```python
from build123d import *

# Parameters (mm, degrees)
PAD015_DEPTH            = 17
SKETCH026_R             = 1.6
POCKET011_DEPTH         = 5
POCKET012_DEPTH         = 5
FILLET004_R             = 1
CHAMFER002_SIZE         = 2
CHAMFER003_SIZE         = 1
PAD014_DEPTH            = 7
FILLET003_R             = 1
FILLET002_R             = 0.4
BODY006_ROLL_ANGLE      = -90
BODY006_PLACEMENT_ANGLE = 180


with BuildPart() as obj1:
    # Sketch027 → Pad015 (new body)
    with BuildSketch(Plane.XY):
        Polygon((-2, -24.6), (-2, -2), (-13, -2), (-13, 0), (0, 0), (0, -22.6), (18.4, -22.6), (18.4, 3.4), (20.4, 3.4), (20.4, -24.6), align=None)
    extrude(amount=PAD015_DEPTH)

    # Sketch026 (on Face2 of Pad015) → Pocket011 (cut)
    with BuildSketch(Plane.XZ.offset(2)):
        with Locations((-9, 3.655766)):
            Circle(SKETCH026_R)
        with Locations((-9, 12.077909)):
            Circle(SKETCH026_R)
    extrude(amount=-POCKET011_DEPTH, mode=Mode.SUBTRACT)

    # Sketch025 → Pocket012 (cut)
    with BuildSketch(Plane(origin=(18.4, 0, 0), x_dir=(0, -1, 0), z_dir=(-1, 0, 0))):
        with BuildLine():
            ThreePointArc((9.9528471273, 16.0383040886), (11.1, 12.4), (12.2471528727, 16.0383040886))
            Line((11.1, 16.8415491775), (12.2471528727, 16.0383040886))
            Line((9.9528471273, 16.0383040886), (11.1, 16.8415491775))
        make_face()
    extrude(amount=-POCKET012_DEPTH, mode=Mode.SUBTRACT)

    # Fillet004
    fillet004_edges = [obj1.edges().sort_by_distance(p)[0] for p in [
        (-2, -24.6, 8.5),
        (20.4, -24.6, 8.5),
    ]]
    fillet(fillet004_edges, radius=FILLET004_R)

    # Chamfer002
    chamfer002_edges = [obj1.edges().sort_by_distance(p)[0] for p in [
        (-13, -1, 17),
        (-13, -1, 0),
    ]]
    chamfer(chamfer002_edges, length=CHAMFER002_SIZE)

    # Chamfer003
    chamfer003_edges = [obj1.edges().sort_by_distance(p)[0] for p in [
        (20.4, 3.4, 8.5),
    ]]
    chamfer(chamfer003_edges, length=CHAMFER003_SIZE)

    # Sketch028 (on Face1 of Chamfer003) → Pad014 (join)
    with BuildSketch(Plane(origin=(0, 0, 0), x_dir=(1, 0, 0), z_dir=(0, 0, -1))):
        Polygon((13.8, 24.6), (12.4, 24.6), (12.4, 26.8), (8, 26.8), (8, 25.6), (6.6, 25.6), (6.6, 28.2), (13.8, 28.2), align=None)
    extrude(amount=-PAD014_DEPTH)

    # Fillet003
    fillet003_edges = [obj1.edges().sort_by_distance(p)[0] for p in [
        (12.4, -24.6, 3.5),
        (13.8, -24.6, 3.5),
    ]]
    fillet(fillet003_edges, radius=FILLET003_R)

    # Fillet002
    fillet002_edges = [obj1.edges().sort_by_distance(p)[0] for p in [
        (13.8, -28.2, 3.5),
        (6.6, -28.2, 3.5),
        (6.6, -25.6, 3.5),
        (12.4, -26.8, 3.5),
        (8, -26.8, 3.5),
        (8, -25.6, 3.5),
    ]]
    fillet(fillet002_edges, radius=FILLET002_R)


with BuildPart() as obj1_1:
    # Body006 roll: moved
    add(obj1.part.rotate(Axis((0, 0, 0), (1, 0, 0)), BODY006_ROLL_ANGLE))


with BuildPart() as obj1_2:
    # Body006 placement: moved
    add(obj1_1.part.moved(Location((-26.5, 36.8, 2.5))).rotate(Axis((-26.5, 36.8, 2.5), (0, 0, 1)), BODY006_PLACEMENT_ANGLE))


with BuildPart() as part_mirroring001:
    # Part__Mirroring001: instance of obj1
    add(obj1_2.part.mirror(Plane(origin=(0, 0, 0), x_dir=(0, -1, 0), z_dir=(1, 0, 0))))


solid = part_mirroring001.part
```
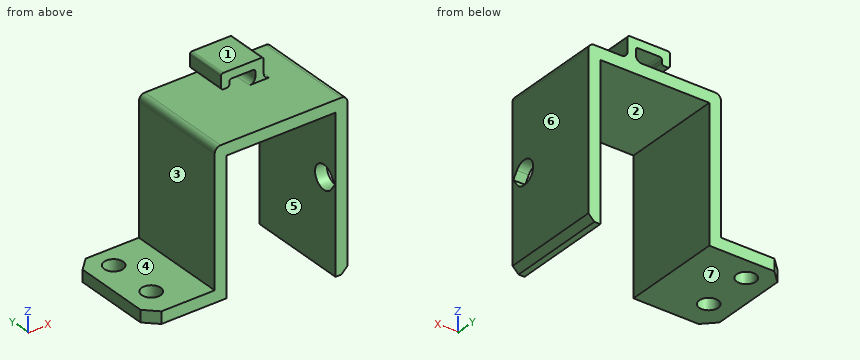
CAD build for the part. Positions are in the model's coordinates, mm. Face numbers are marked on the shaded views. A direction names the side the tool comes from. Coordinates: 2 decimals unless noted, no trailing zeros. Write each loop counter-clockwise with the first axis right and the second up, starting at its lowest first coordinate (ties: lowest second). Pieces come first, ordered by that corner, then holes. Notation, with made-up numbers: (51.5, 74) -> (83.5, 74) arc R35 ccw to (83.5, 110) -> close; hole circle Ø8 at (71, 84.25). An arc over 180 degrees is marked (long way). Return JSON: item names as keys, results as strings. Group by question number.
Q1. Cut at A-A, the plane x = 17.5. Give the cut face in (y, z), then the cut area to 3 significant figures.
Q2. Which spindle directions (+Z, -Z, +X, -X, +Y, -Y) get a long thin tool onto all of the face, cutting with end or side? Do the marked faces 4, 5, 6 and 7. Say none if no direction does.
Q3. Cut at C-C, the plane z = 16. Give the cut face in (x, y).
Q4. Cut at B-B, the plane y = 22.4. Give the cut face in (x, z), then the cut area to 3 significant figures.
Q5. Pull direction X, two halves, no side cores. Call the marked faces 1, 2 and 3: released by +X, released by -X, zero draft, split by the parting line, or undercut.
Q6. Flat gauge pins, fed straight in: pin 1 (5 mm diameter, centred on x = 31.5, y = 30.5, fed in from -Z); pin 2 (0.7 mm diameter, centred on y = 32, z = 29, fed in from +X); pin 3 (5 mm diameter, centred on x = 20.5, y = 29.5, fed in from +Z). Where does each tip first touch, or does it go through?
Q7. Drill centre lines: line 1 (X direction, y = 34.25, z = 15.5); line 2 (Y direction, x = 17, z = 3); line 3 (Z direction, x = 36.5, y = 32.25). Where is each one in solid material? Low to high.
Returned:
{
 "1": {"outline": "(19.8, 2.5) -> (23.12, 2.5) -> (23.12, 4.5) -> (19.8, 4.5) -> close; (26.32, 2.5) -> (31.54, 2.5) -> (31.54, 4.5) -> (26.32, 4.5) -> close; (34.74, 2.5) -> (36.8, 2.5) -> (36.8, 4.5) -> (34.74, 4.5) -> close", "area": "21.2 mm2"},
 "2": {"face 4": "+Z, -X, +Y, -Y", "face 5": "-Z, +Y, -Y", "face 6": "+Z, -Z, +X, +Y, -Y", "face 7": "-Z, -X, +Y, -Y"},
 "3": {"outline": "(24.5, 19.8) -> (26.5, 19.8) -> (26.5, 36.8) -> (24.5, 36.8) -> close; (44.9, 19.8) -> (46.9, 19.8) -> (46.9, 36.8) -> (44.9, 36.8) -> close"},
 "4": {"outline": "(13.5, 2.5) -> (26.5, 2.5) -> (26.5, 25.1) -> (44.9, 25.1) -> (44.9, 15.6) -> (46.9, 15.6) -> (46.9, 26.1) arc R1 ccw to (45.9, 27.1) -> (25.5, 27.1) arc R1 ccw to (24.5, 26.1) -> (24.5, 4.5) -> (13.5, 4.5) -> close; (44.9, -0.9) -> (45.9, -0.9) -> (46.9, 0.1) -> (46.9, 11.6) -> (44.9, 11.6) -> close", "area": "155 mm2"},
 "5": {"face 1": "zero draft", "face 2": "undercut", "face 3": "released by -X"},
 "6": {"pin 1": "stops at z = 25.1", "pin 2": "stops at x = 40.3", "pin 3": "stops at z = 4.5"},
 "7": {"line 1": "x = 24.5 to 26.5, 44.9 to 46.9", "line 2": "y = 19.8 to 23.2, 26.24 to 31.62, 34.66 to 36.8", "line 3": "z = 25.1 to 27.1, 29.3 to 30.7"}
}
